Geometry: final body of the model. Coordinates: model frame, mm. Face numbers are marked on the shaded views. A direction names the side the tool comes from. Give positions to 0.01 mm unless a question says otherwise; leave off trailing zeros. Write each loop counter-clockwise with the first axis right and the second up, starting at its lowest first coordinate (ties: lowest second). Pieces come first, ordered by that corner, then holes.
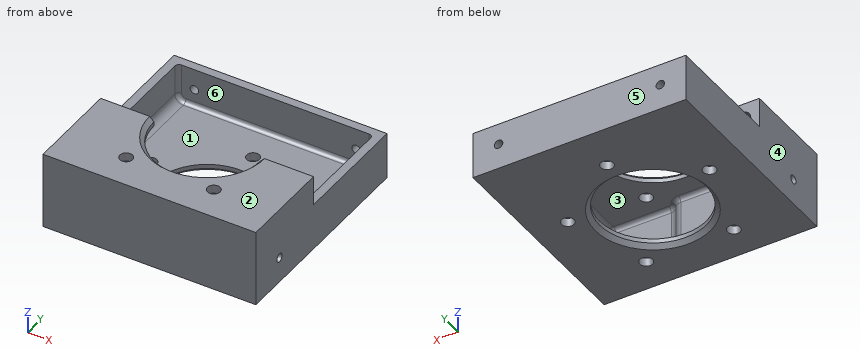
from build123d import *

# Parameters (mm, degrees)
SKETCH1_W          = 50
SKETCH1_H          = 50
MAIN_DEPTH         = 18
SKETCH2_W          = 7
SKETCH2_H          = 28
CUT_EXTRUDE1_DEPTH = 73.965745388
SHELL1_T           = -2
RIB1_REACH         = 72.285
SKETCH11_WALLS_W   = 12
SKETCH11_WALLS_H   = 158.570267126
SKETCH3_R          = 12.5
CUT_EXTRUDE2_DEPTH = 73.965745388
CHAMFER1_SIZE      = 1
CUT_EXTRUDE3_REACH = 74.966
SKETCH4_R          = 1
SKETCH6_R          = 1
CUT_EXTRUDE4_DEPTH = 73.965745388
CUT_EXTRUDE7_REACH = 74.966
SKETCH9_R          = 1.5
CIRPATTERN1_COUNT  = 5
CUT_EXTRUDE8_REACH = 74.966
SKETCH13_R         = 1.5
FILLET1_R          = 2
FILLET2_R          = 2
FILLET4_R          = 2
FILLET5_R          = 2
FILLET6_R          = 2
FILLET3_R          = 1


with BuildPart() as part:
    # Sketch1 → main (new body)
    with BuildSketch(Plane.XY):
        with Locations((25, 25)):
            Rectangle(SKETCH1_W, SKETCH1_H)
    extrude(amount=MAIN_DEPTH)

    # Sketch2 → Cut-Extrude1 (cut, through all)
    with BuildSketch(Plane(origin=(50, 0, 0), x_dir=(0, 0, -1), z_dir=(1, 0, 0))):
        with Locations((-14.5, 36)):
            Rectangle(SKETCH2_W, SKETCH2_H)
    extrude(amount=-CUT_EXTRUDE1_DEPTH, mode=Mode.SUBTRACT)

    # Shell1
    shell1_openings = [part.faces().sort_by_distance(p)[0] for p in [
        (25, 36, 11),
        (25, 22, 14.5),
    ]]
    offset(amount=SHELL1_T, openings=shell1_openings, kind=Kind.INTERSECTION)

    # Sketch11 walls → Rib1 (add, up to next)
    with BuildSketch(Plane(origin=(0, 4, 0), x_dir=(-1, 0, 0), z_dir=(0, 1, 0)), mode=Mode.PRIVATE) as rib1_sk1:
        with Locations((-25, 8)):
            Rectangle(SKETCH11_WALLS_W, SKETCH11_WALLS_H)
    rib1_tool1 = extrude(rib1_sk1.sketch, amount=-RIB1_REACH, mode=Mode.PRIVATE) - part.part
    add(rib1_tool1.solids().sort_by_distance((25, 4, 8))[0])

    # Sketch3 → Cut-Extrude2 (cut, through all)
    with BuildSketch(Plane.XY.offset(18)):
        with Locations((25, 22)):
            Circle(SKETCH3_R)
    extrude(amount=-CUT_EXTRUDE2_DEPTH, mode=Mode.SUBTRACT)

    # Chamfer1
    chamfer1_edges = [part.edges().sort_by_distance(p)[0] for p in [
        (12.5, 22, 0),
        (25, 9.5, 18),
    ]]
    chamfer(chamfer1_edges, length=CHAMFER1_SIZE)

    # Sketch4 → Cut-Extrude3 (cut, up to next)
    with BuildSketch(Plane(origin=(0, 50, 0), x_dir=(-1, 0, 0), z_dir=(0, 1, 0)), mode=Mode.PRIVATE) as cut_extrude3_sk1:
        with Locations((-44, 6)):
            Circle(SKETCH4_R)
    cut_extrude3_tool1 = extrude(cut_extrude3_sk1.sketch, amount=-CUT_EXTRUDE3_REACH, mode=Mode.PRIVATE) & part.part
    # Sketch4 → Cut-Extrude3 (cut, up to next)
    with BuildSketch(Plane(origin=(0, 50, 0), x_dir=(-1, 0, 0), z_dir=(0, 1, 0)), mode=Mode.PRIVATE) as cut_extrude3_sk2:
        with Locations(Location((-6, 6, 0), (0, 0, 180))):
            Circle(SKETCH4_R)
    cut_extrude3_tool2 = extrude(cut_extrude3_sk2.sketch, amount=-CUT_EXTRUDE3_REACH, mode=Mode.PRIVATE) & part.part
    add(cut_extrude3_tool1.solids().sort_by_distance((44, 50, 6))[0], mode=Mode.SUBTRACT)
    add(cut_extrude3_tool2.solids().sort_by_distance((6, 50, 6))[0], mode=Mode.SUBTRACT)

    # Sketch6 → Cut-Extrude4 (cut, through all)
    with BuildSketch(Plane(origin=(50, 0, 0), x_dir=(0, 0, -1), z_dir=(1, 0, 0))):
        with Locations(Location((-6, 9, 0), (0, 0, 90))):
            Circle(SKETCH6_R)
    extrude(amount=-CUT_EXTRUDE4_DEPTH, mode=Mode.SUBTRACT)

    # Sketch9 → Cut-Extrude7 (cut, up to next)
    with BuildSketch(Plane(origin=(0, 0, 0), x_dir=(-1, 0, 0), z_dir=(0, 0, -1)), mode=Mode.PRIVATE) as cut_extrude7_sk1:
        with Locations((-25, 39.5)):
            Circle(SKETCH9_R)
    cut_extrude7_tool1 = extrude(cut_extrude7_sk1.sketch, amount=-CUT_EXTRUDE7_REACH, mode=Mode.PRIVATE) & part.part
    cut_extrude7 = cut_extrude7_tool1.solids().sort_by_distance((25, 39.5, 0))[0]
    add(cut_extrude7, mode=Mode.SUBTRACT)

    # CirPattern1: Cut-Extrude7 ×5 about axis
    cirpattern1_axis = Axis((25, 22, 0), (0, 0, 1))
    for i in range(1, CIRPATTERN1_COUNT):
        add(cut_extrude7.rotate(cirpattern1_axis, i * 360 / CIRPATTERN1_COUNT), mode=Mode.SUBTRACT)

    # Sketch13 → Cut-Extrude8 (cut, up to next)
    with BuildSketch(Plane.XY.offset(18), mode=Mode.PRIVATE) as cut_extrude8_sk1:
        with Locations(Location((35.286241915, 7.842202598, 0), (0, 0, 180))):
            Circle(SKETCH13_R)
    cut_extrude8_tool1 = extrude(cut_extrude8_sk1.sketch, amount=-CUT_EXTRUDE8_REACH, mode=Mode.PRIVATE) & part.part
    # Sketch13 → Cut-Extrude8 (cut, up to next)
    with BuildSketch(Plane.XY.offset(18), mode=Mode.PRIVATE) as cut_extrude8_sk2:
        with Locations(Location((14.713758085, 7.842202598, 0), (0, 0, 180))):
            Circle(SKETCH13_R)
    cut_extrude8_tool2 = extrude(cut_extrude8_sk2.sketch, amount=-CUT_EXTRUDE8_REACH, mode=Mode.PRIVATE) & part.part
    add(cut_extrude8_tool1.solids().sort_by_distance((35.286242, 7.842203, 18))[0], mode=Mode.SUBTRACT)
    add(cut_extrude8_tool2.solids().sort_by_distance((14.713758, 7.842203, 18))[0], mode=Mode.SUBTRACT)

    # Fillet1
    fillet1_edges = [part.edges().sort_by_distance(p)[0] for p in [
        (2, 12, 16),
        (48, 12, 16),
        (2, 25, 2),
        (48, 25, 2),
    ]]
    fillet(fillet1_edges, radius=FILLET1_R)

    # Fillet2
    fillet2_edges = [part.edges().sort_by_distance(p)[0] for p in [
        (31, 2, 9),
    ]]
    fillet(fillet2_edges, radius=FILLET2_R - 0.0001)  # a hair under: the kernel refuses the full size

    # Fillet4
    fillet4_edges = [part.edges().sort_by_distance(p)[0] for p in [
        (31, 4, 9),
    ]]
    fillet(fillet4_edges, radius=FILLET4_R)

    # Fillet5
    fillet5_edges = [part.edges().sort_by_distance(p)[0] for p in [
        (19, 4, 9),
    ]]
    fillet(fillet5_edges, radius=FILLET5_R - 0.0001)  # a hair under: the kernel refuses the full size

    # Fillet6
    fillet6_edges = [part.edges().sort_by_distance(p)[0] for p in [
        (19, 2, 9),
    ]]
    fillet(fillet6_edges, radius=FILLET6_R)

    # Fillet3
    fillet3_edges = [part.edges().sort_by_distance(p)[0] for p in [
        (48, 2, 9),
        (47.414213562, 2, 15.414213562),
        (47.414213562, 2, 2.585786438),
        (10.76792806, 2, 2),
        (25, 48, 2),
        (2.585786438, 48, 2.585786438),
        (47.414213562, 48, 2.585786438),
        (10.76792806, 2, 16),
        (2, 2, 9),
        (2.585786438, 2, 2.585786438),
        (2.585786438, 2, 15.414213562),
        (39.49995, 2, 2),
        (39.49995, 2, 16),
        (31.9999375, 2.267943012, 16),
        (31.9999375, 2.267943012, 2),
        (30.535868621, 3.73204359, 2),
        (30.535868621, 3.73204359, 16),
        (25.26787806, 4, 16),
        (25.26787806, 4, 2),
        (19.9999375, 3.732056988, 16),
        (19.9999375, 3.732056988, 2),
        (18.535868621, 2.26795641, 16),
        (18.535868621, 2.26795641, 2),
        (2, 48, 7.5),
        (48, 48, 7.5),
    ]]
    fillet(fillet3_edges, radius=FILLET3_R)


solid = part.part
Q1. Section B-B on x = 44. Output: boundary loops of the cut face in (y, z), plus the area to 3 significant figures.
Filled sheet:
outline: (0, 0) - (50, 0) - (50, 5) - (48, 5) - (48, 3) arc R1 cw to (47, 2) - (3, 2) arc R1 cw to (2, 3) - (2, 15) arc R1 cw to (3, 16) - (22, 16) - (22, 18) - (0, 18) - close; (48, 7) - (50, 7) - (50, 11) - (48, 11) - close
area: 187 mm2
Q2. Section C-C on z = 6. Count the separate pieces of the cut face and the enclosed holes in it, plus the area to 3 significant figures.
Filled sheet:
separate pieces: 4
enclosed holes: 0
area: 393 mm2
Q3. Ray query, line 1 along Y through (x, z) = (25, 1.45); line 2 along Z through (x, y) = (44, 49.35); line 3 along X through (y, z) = (21, 13.5). Return the intervals inside material, ascending.
Filled sheet:
line 1: y = 0 to 9.5, 34.5 to 38, 41 to 50
line 2: z = 0 to 5, 7 to 11
line 3: x = 0 to 2, 48 to 50
Q4. Pin query (flat end, axial travel): P1, Ø8, axis at x = 7, y = 34.5, coming from the -Z side; P2, Ø1.6, axis at x = 44, z = 6, coming from the +Y side; P3, Ø10, axis at x = 14.5, y = 28, coming from the +Z side; P4, Ø5.5, axis at x = 45, z = 14, coming from the +Y side. Return the tip coordinate at first contact, or that it passes through.
Filled sheet:
P1: stops at z = 0
P2: stops at y = 2
P3: stops at z = 2
P4: stops at y = 22
Q5. Section A-A on y = 39.5. Output: boundary loops of the cut face in (x, z), plus the area to 3 significant figures.
Filled sheet:
outline: (0, 0) - (23.5, 0) - (23.5, 2) - (4, 2) arc R2 cw to (2, 4) - (2, 11) - (0, 11) - close; (26.5, 0) - (50, 0) - (50, 11) - (48, 11) - (48, 4) arc R2 cw to (46, 2) - (26.5, 2) - close
area: 132 mm2
Q6. Pull-direction query (X, two-part tool) for the marked faces 4, 5 and 6; classes: released by +X, released by -X, zero draft, split by the parting line, or undercut.
Filled sheet:
face 4: released by -X
face 5: zero draft
face 6: undercut
Q7. Access query for the marked faces 1, 2 and 3. Directions: +Z, -Z, +X, -X, +Y, -Y. A direction counts if a zero-diameter tool reaches every point of the face in a straight line with its end or side. Return the directions, or none.
Filled sheet:
face 1: none
face 2: +Z, +X, -X, +Y, -Y
face 3: +Y
